Geometry check sheet. Reference: the model listing, model coordinates, mm. A direction names the side the tool comes from. Coordinates: 2 decimals unless noted, no trailing zeros. Write each loop counter-clockwise with the first axis right and the second up, starting at its lowest first coordinate (ties: lowest second). Pieces come first, ordered by that corner, then holes. Notation, with made-up numbers: (22.5, 65) -> (62.5, 65) arc R18 cw to (62.5, 71) -> close; hole circle Ø4 at (15, 45.5). An arc over 180 degrees is marked (long way). Put each result on its own line as item: value. Start each with the question number.
from build123d import *

# Parameters (mm, degrees)
SKETCH1_W           = 30
SKETCH1_H           = 17.96
BOSS_EXTRUDE1_DEPTH = 30
SKETCH2_R           = 14
CUT_EXTRUDE1_DEPTH  = 2
SKETCH3_R           = 1.7
CUT_EXTRUDE2_DEPTH  = 2
SKETCH4_R           = 9
CUT_EXTRUDE3_DEPTH  = 2
SKETCH5_R           = 3
CUT_EXTRUDE6_DEPTH  = 90.858350753
CUT_EXTRUDE7_DEPTH  = 2
BOSS_EXTRUDE2_DEPTH = 1
EXTRUDE_THIN1_DEPTH = 0.7


with BuildPart() as part:
    # Sketch1 → Boss-Extrude1 (new body)
    with BuildSketch(Plane.XY):
        with Locations((15, 8.98)):
            Rectangle(SKETCH1_W, SKETCH1_H)
        Polygon((30, 17.96), (30, 0), (53.04, 0), (53.04, 80), (30, 80), align=None)
    extrude(amount=BOSS_EXTRUDE1_DEPTH)

    # Sketch2 → Cut-Extrude1 (cut)
    with BuildSketch(Plane(origin=(0, 17.96, 0), x_dir=(1, 0, 0), z_dir=(0, 1, 0))):
        with Locations(Location((15, -15.240313603, 0), (0, 0, 270))):
            Circle(SKETCH2_R)
    extrude(amount=-CUT_EXTRUDE1_DEPTH, mode=Mode.SUBTRACT)

    # Sketch3 → Cut-Extrude2 (cut)
    with BuildSketch(Plane(origin=(0, 15.96, 0), x_dir=(1, 0, 0), z_dir=(0, 1, 0))):
        with Locations(Location((15, -3.4, 0), (0, 0, 270))):
            Circle(SKETCH3_R)
        with Locations(Location((26.6, -14.898975901, 0), (0, 0, 270))):
            Circle(SKETCH3_R)
        with Locations(Location((14.997277846, -26.6, 0), (0, 0, 270))):
            Circle(SKETCH3_R)
        with Locations(Location((3.4, -15.0181958, 0), (0, 0, 270))):
            Circle(SKETCH3_R)
    extrude(amount=-CUT_EXTRUDE2_DEPTH, mode=Mode.SUBTRACT)

    # Sketch4 → Cut-Extrude3 (cut)
    with BuildSketch(Plane(origin=(0, 15.96, 0), x_dir=(1, 0, 0), z_dir=(0, 1, 0))):
        with Locations(Location((15, -15.240313603, 0), (0, 0, 270))):
            Circle(SKETCH4_R)
    extrude(amount=-CUT_EXTRUDE3_DEPTH, mode=Mode.SUBTRACT)

    # Sketch5 → Cut-Extrude6 (cut, through all)
    with BuildSketch(Plane(origin=(0, 13.96, 0), x_dir=(1, 0, 0), z_dir=(0, 1, 0))):
        with Locations(Location((15, -15.240313603, 0), (0, 0, 270))):
            Circle(SKETCH5_R)
    extrude(amount=-CUT_EXTRUDE6_DEPTH, mode=Mode.SUBTRACT)

    # Sketch6 → Cut-Extrude7 (cut)
    with BuildSketch(Plane.ZY.offset(-30)):
        with BuildLine():
            Line((4.639681938, 75.339266158), (4.639681938, 30.209714413))
            ThreePointArc((4.639681938, 30.209714413), (6.339681938, 28.509714413), (8.039681938, 30.209714413))
            Line((8.039681938, 30.209714413), (8.039681938, 75.339266158))
            ThreePointArc((8.039681938, 75.339266158), (6.339681938, 77.039266158), (4.639681938, 75.339266158))
        make_face()
        with BuildLine():
            Line((21.70723863, 75.339266158), (21.70723863, 30.209714413))
            ThreePointArc((21.70723863, 30.209714413), (23.40723863, 28.509714413), (25.10723863, 30.209714413))
            Line((25.10723863, 30.209714413), (25.10723863, 75.339266158))
            ThreePointArc((25.10723863, 75.339266158), (23.40723863, 77.039266158), (21.70723863, 75.339266158))
        make_face()
    extrude(amount=-CUT_EXTRUDE7_DEPTH, mode=Mode.SUBTRACT)

    # Sketch7 → Boss-Extrude2 (add)
    with BuildSketch(Plane(origin=(0, 0, 0), x_dir=(-1, 0, 0), z_dir=(0, 0, -1))):
        Polygon((-15, 17.96), (-30, 29.475844043), (-30, 17.96), align=None)
    extrude(amount=-BOSS_EXTRUDE2_DEPTH)

    # Sketch8 → Extrude-Thin1 (add)
    with BuildSketch(Plane.XY.offset(30)):
        Polygon((15, 17.96), (30, 29.475844043), (36.089590867, 21.543827713), (21.089590867, 10.027983669), align=None)
    extrude(amount=-EXTRUDE_THIN1_DEPTH)


solid = part.part
Item 1: Section check A-A, the plane y = 36. Enter the section's corners in (x, z).
Item 2: Access from +Z, -Z, +X, -X, +Y, -Y to the whole of each face (thin tool, end or side, straight path). Record for faces 1 (the cylindrical face through (12.07, 7.08, 14.59)), 2 (the flat face through (31, 52, 25.107)), 3 (the flat face through (30, 49, 15)), 4 (the flat face through (15, 13.96, 3)), 5 (the flat face through (22.4, 23.64, 0.49)).
Item 3: Mould release check, pull along Z, two halves, no side actions. Record for faces 6 (the flat face through (26, 0, 15)), 7 (the flat face through (33, 32, 0)), 8 (the flat face through (32, 53, 23)): released by +Z, released by -Z, zero draft, split by the parting line, or undercut.
Item 4: Section check B-B, the plane z = 14.5. Enter the section's corners in (x, y).
Item 5: Go/stop test with flat-tipped pins: P1, Ø9, axis at x = 21.5, y = 22.5, coming from the -Z side; P2, Ø2, axis at x = 12.5, z = 22.5, coming from the +Y side; P3, Ø3.5, axis at y = 54, z = 23.5, coming from the -X side; P4, Ø5.5, axis at x = 3.4, z = 15.02, coming from the +Y side. Record where each tip stops, or that it passes through.
Item 6: Section check C-C, the plane z = 3.4. Enter the section's corners in (x, y), and give its area (3 significant figures).
Item 7: Scan lines: line 1 along X through (y, z) = (56, 23.25); line 2 along Y through (x, z) = (8.5, 5.5); line 3 along X through (y, z) = (15.15, 26.6). Record each from-to range of solid material in increasing order. Write a range as [from, to].
Item 8: Section check D-D, the plane x = 20. Enter the section's corners in (y, z).
From the geometry:
1. outline: (30, 0) -> (53.04, 0) -> (53.04, 30) -> (30, 30) -> (30, 25.11) -> (32, 25.11) -> (32, 21.71) -> (30, 21.71) -> (30, 8.04) -> (32, 8.04) -> (32, 4.64) -> (30, 4.64) -> close
2. face 1: +Y, -Y
2. face 2: -X
2. face 3: -X, +Y
2. face 4: +Y
2. face 5: +Z, -Z, -X, +Y
3. face 6: zero draft
3. face 7: released by -Z
3. face 8: undercut
4. outline: (0, 0) -> (12.09, 0) -> (12.09, 13.96) -> (6.03, 13.96) -> (6.03, 15.96) -> (5.02, 15.96) -> (5.02, 13.96) -> (1.78, 13.96) -> (1.78, 15.96) -> (1.02, 15.96) -> (1.02, 17.96) -> (0, 17.96) -> close; (17.91, 0) -> (53.04, 0) -> (53.04, 80) -> (30, 80) -> (30, 17.96) -> (28.98, 17.96) -> (28.98, 15.96) -> (28.25, 15.96) -> (28.25, 13.96) -> (24.95, 13.96) -> (24.95, 15.96) -> (23.97, 15.96) -> (23.97, 13.96) -> (17.91, 13.96) -> close
5. P1: z = 0
5. P2: y = 13.96
5. P3: x = 30
5. P4: y = 17.96
6. outline: (0, 0) -> (53.04, 0) -> (53.04, 80) -> (30, 80) -> (30, 17.96) -> (22.47, 17.96) -> (22.47, 15.96) -> (16.7, 15.96) -> (16.7, 13.96) -> (13.3, 13.96) -> (13.3, 15.96) -> (7.53, 15.96) -> (7.53, 17.96) -> (0, 17.96) -> close
6. area: 2,350 mm²
7. line 1: [32, 53.04]
7. line 2: [0, 15.96]
7. line 3: [0, 13.3], [16.7, 53.04]
8. outline: (0, 0) -> (21.8, 0) -> (21.8, 1) -> (17.96, 1) -> (17.96, 2.16) -> (15.96, 2.16) -> (15.96, 7.76) -> (13.96, 7.76) -> (13.96, 22.72) -> (15.96, 22.72) -> (15.96, 28.32) -> (17.96, 28.32) -> (17.96, 29.3) -> (21.8, 29.3) -> (21.8, 30) -> (0, 30) -> close
